CAD build for the part. Positions are in the model's coordinates, mm. A direction names the side the tool comes from. Round coordinates to 2 decimals unless told otherwise and drop trailing zeros. Loops run counter-clockwise (first coordinate to the right, second up) from the corner with the lowest first, then second, coordinate; pieces in that order, holes last. Notation, with made-up numbers: M 72.5,24.25 L 85.5,24.25 A28 cw 85.5,44.25 Z; hole C 14,78 d8. An arc over 180 degrees is marked long. Use one line per item in the form item = value.
from build123d import *

# Parameters (mm, degrees)
F2_R = 5.99999


# Not quite as in the source:
# - a fillet or chamfer is up to 0.001 mm smaller than in the source, because OpenCascade refuses the exact size


with BuildPart() as f1:
    # F0 (on Top) → F1 (revolve)
    with BuildSketch(Plane.XY):
        with BuildLine():
            Line((-32.2816833258, 6), (25.7183166742, 6))
            Line((25.7183166742, 6), (25.7183166742, 16))
            Line((25.7183166742, 16), (22.7183166742, 16))
            Line((22.7183166742, 16), (22.7183166742, 20))
            Line((22.7183166742, 20), (5.7183166742, 20))
            Line((5.7183166742, 20), (5.7183166742, 31))
            Line((5.7183166742, 31), (-6.2816833258, 31))
            ThreePointArc((-6.2816833258, 31), (-12.2816833258, 25.0169717373), (-18.2816833258, 31))
            Line((-18.2816833258, 31), (-62.2816833258, 31))
            Line((-62.2816833258, 31), (-62.2816833258, 25))
            Line((-62.2816833258, 25), (-60.7816833258, 25))
            Line((-60.7816833258, 25), (-60.7816833258, 16))
            Line((-60.7816833258, 16), (-48.7816833258, 16))
            Line((-48.7816833258, 16), (-48.7816833258, 13.4885394946))
            Line((-48.7816833258, 13.4885394946), (-45.7816833258, 13.4885394946))
            Line((-45.7816833258, 13.4885394946), (-45.7816833258, 20.5))
            Line((-45.7816833258, 20.5), (-40.2816833258, 20.5))
            Line((-40.2816833258, 20.5), (-40.2816833258, 16))
            Line((-40.2816833258, 16), (-32.2816833258, 16))
            Line((-32.2816833258, 16), (-32.2816833258, 6))
        make_face()
    revolve(axis=Axis((-40.0854273438, 0, 0), (1, 0, 0)))

    # F2 (radius 6 in the source; OpenCascade refuses exactly that, so slightly less here)
    f2_edges = [f1.edges().sort_by_distance(p)[0] for p in [
        (-62.281683, -31, 0),
    ]]
    fillet(f2_edges, radius=F2_R)


solid = f1.part
1. Pull direction Y, two halves, no side cores. Call faces 6 (the face through (-60.782, -0.3, -16.3)), 7 (the face through (-37.548, -4.036, 30.736)), 8 (the face through (22.718, 8.98, 13.43)): +Y half, -Y half, draft (parallel to the pull), parting line (faces both ways), or undercut.
Completed:
face_6 = undercut
face_7 = parting line
face_8 = draft
2. Tool access for faces 1 (the face through (-40.282, 12, -11)), 2 (the face through (24.2, -3.47, -15.62)), 3 (the face through (-47.261, -1.756, 13.374)), 4 (the face through (-0.366, -4.036, 30.736)), 5 (the face through (25.718, -7, 0)): list every direction of +Z, -Z, +X, -X, +Y, -Y with a clear straight run to the whole face (end or side of a thin tool).
Completed:
face_1 = none
face_2 = +X
face_3 = -X
face_4 = +X, -X
face_5 = +Z, -Z, +X, +Y, -Y
3. Drop flat-ended pins along their axis: P1, Ø2, axis at x = -21.5, z = -18.5, coming from the -Y side; P2, Ø24.5, axis at y = 0, z = 0, coming from the -X side; P3, Ø8, axis at y = 15.5, z = 22.5, coming from the +X side; P4, Ø9.5, axis at y = 0, z = 0, coming from the +X side. Give the stop position or say it passes through.
Completed:
P1 = -25.59
P2 = -32.28
P3 = 5.72
P4 = through
4. Cut at B-B on x = -1.5. Write the cut outline in (y, z), and give its area (3 significant figures).
Completed:
outline = C 0,0 d62; hole C 0,0 d12
area = 2,910 mm2
5. Cut at A-A on x = 15.5. Write the cut outline in (y, z).
Completed:
outline = C 0,0 d40; hole C 0,0 d12
6. Probe line 1 along Z through (x, y) = (-47.35, 0); line 2 along Z through (x, y) = (-35.5, 0); line 3 along X through (y, z) = (11.5, 14). List the from-to ranges inside material, lowest first. Write a range as from..to.
Completed:
line_1 = -31..-13.49, 13.49..31
line_2 = -31..-16, 16..31
line_3 = -60.78..-45.78, -40.28..22.72
